```python
from build123d import *

# Parameters (mm, degrees)
SKETCH_R        = 2.8
SKETCH_R_2      = 4.3
PAD_DEPTH       = 21.5
SKETCH001_R     = 4.5
POCKET_DEPTH    = 6
SKETCH002_R     = 6.6
POCKET001_DEPTH = 9
FILLET_R        = 4


with BuildPart() as part:
    # Sketch → Pad (new body)
    with BuildSketch(Plane.XY):
        with BuildLine():
            Line((0, 0), (50, 0))
            Line((50, 0), (63.325334, 10.29541))
            ThreePointArc((63.325334, 10.29541), (67.6, 19), (63.325334, 27.70459))
            Line((50, 38), (63.325334, 27.70459))
            Line((50, 38), (0, 38))
            Line((0, 38), (-13.325334, 27.70459))
            ThreePointArc((-13.325334, 27.70459), (-17.6, 19), (-13.325334, 10.29541))
            Line((0, 0), (-13.325334, 10.29541))
        make_face()
        with Locations((5, 31)):
            Circle(SKETCH_R, mode=Mode.SUBTRACT)
        with Locations((45, 31)):
            Circle(SKETCH_R, mode=Mode.SUBTRACT)
        with Locations((45, 7)):
            Circle(SKETCH_R, mode=Mode.SUBTRACT)
        with Locations((5, 7)):
            Circle(SKETCH_R, mode=Mode.SUBTRACT)
        with Locations((-6.6, 19)):
            Circle(SKETCH_R_2, mode=Mode.SUBTRACT)
        with Locations((56.6, 19)):
            Circle(SKETCH_R_2, mode=Mode.SUBTRACT)
    extrude(amount=PAD_DEPTH)

    # Sketch001 (on Face16 of Pad) → Pocket (cut)
    with BuildSketch(Plane.XY.offset(21.5)):
        with Locations((5, 31)):
            Circle(SKETCH001_R)
        with Locations((45, 31)):
            Circle(SKETCH001_R)
        with Locations((45, 7)):
            Circle(SKETCH001_R)
        with Locations((5, 7)):
            Circle(SKETCH001_R)
    extrude(amount=-POCKET_DEPTH, mode=Mode.SUBTRACT)

    # Sketch002 (on Face4 of Pocket) → Pocket001 (cut)
    with BuildSketch(Plane(origin=(0, 0, 0), x_dir=(1, 0, 0), z_dir=(0, 0, -1))):
        with Locations((-6.6, -19)):
            Circle(SKETCH002_R)
        with Locations((56.6, -19)):
            Circle(SKETCH002_R)
    extrude(amount=-POCKET001_DEPTH, mode=Mode.SUBTRACT)

    # Fillet
    fillet_edges = [part.edges().sort_by_distance(p)[0] for p in [
        (0, 38, 10.75),
        (0, 0, 10.75),
        (50, 0, 10.75),
        (50, 38, 10.75),
    ]]
    fillet(fillet_edges, radius=FILLET_R)


solid = part.part
```
CAD build for the part. Positions are in the model's coordinates, mm. A direction names the side the tool comes from. Round coordinates to 2 decimals unless told otherwise and drop trailing zeros. Order: outer loops, then holes, each group sorted by start corner. A loop starts at its lowest first (then second) coordinate and runs counter-clockwise, first axis right, second up. Notation, with made-up numbers: (40, 55.25) - (51, 55.25) arc R23 cw to (51, 69.25) - close; hole circle Ø6 at (74, 72). An arc over 180 degrees is marked (long way). Use CSV: the item, a comma, the result in double quotes. Start each with the question number.
1) Saw through at B-B (y = 31). List the corners of the cut face in (x, z), and give its area (3 significant figures).
2) Saw through at D-D (x = 56.6). List the corners of the cut face in (y, z), and give its area (3 significant figures).
3) Saw through at A-A (z = 13.5). List the corners of the cut face in (x, y).
4) Wall check: L1, parallel to Y at x = 45, z = 7.5; L2, parallel to X at y = 19, z = 4.75; L3, parallel to X at y = 7, z = 9. Give the ranges that are in metal, low to high. Write a range as [from, to].
5) Two-plate mould, pull along Y, no slides. Class faces 4 (the cylindrical face through (4.02, 26.61, 18.54)), 5 (the flat face through (24, 19, 21.5)), 6 (the flat face through (-7.12, 5.5, 10.6)): pulls with the +Y half, pulls with the -Y half, needs draft (parallel to the pull), parting line crosses it, or undercut.
6) Pin check, flat tips, straight feed: pin 1 Ø2.5 at (x, y) = (5.5, 32.5) entering from +Z; pin 2 Ø10 at (x, z) = (-5.5, 6) entering from +Y; pin 3 Ø1 at (x, z) = (-8, 6) entering from -Y. Stop position of each tip, or through.
7) Saw through at C-C (x = 45). List the corners of the cut face in (y, z).
8) Tool access for faces 1 (the cylindrical face through (-0.503, 21.528, 4.437)), 2 (the flat face through (45, 4, 15.5)), 3 (the cylindrical face through (-2.5, 20.3, 15.2)): list every direction of +Z, -Z, +X, -X, +Y, -Y with a clear straight run to the whole face (end or side of a thin tool).
Values follow:
1,outline,"(-9.06, 0) - (2.2, 0) - (2.2, 15.5) - (0.5, 15.5) - (0.5, 21.5) - (-9.06, 21.5) - close; (7.8, 0) - (42.2, 0) - (42.2, 15.5) - (40.5, 15.5) - (40.5, 21.5) - (9.5, 21.5) - (9.5, 15.5) - (7.8, 15.5) - close; (47.8, 0) - (59.06, 0) - (59.06, 21.5) - (49.5, 21.5) - (49.5, 15.5) - (47.8, 15.5) - close"
1,area,"1,180 mm2"
2,outline,"(5.1, 0) - (12.4, 0) - (12.4, 9) - (14.7, 9) - (14.7, 21.5) - (5.1, 21.5) - close; (23.3, 9) - (25.6, 9) - (25.6, 0) - (32.9, 0) - (32.9, 21.5) - (23.3, 21.5) - close"
2,area,"371 mm2"
3,outline,"(-13.33, 10.3) - (-1.08, 0.83) arc R4 ccw to (1.37, 0) - (48.63, 0) arc R4 ccw to (51.08, 0.83) - (63.33, 10.3) arc R11 ccw to (63.33, 27.7) - (51.08, 37.17) arc R4 ccw to (48.63, 38) - (1.37, 38) arc R4 ccw to (-1.08, 37.17) - (-13.33, 27.7) arc R11 ccw to start; hole circle Ø8.6 at (-6.6, 19); hole circle Ø5.6 at (5, 7); hole circle Ø5.6 at (5, 31); hole circle Ø5.6 at (45, 7); hole circle Ø5.6 at (45, 31); hole circle Ø8.6 at (56.6, 19)"
4,L1,"y = [0, 4.2], [9.8, 28.2], [33.8, 38]"
4,L2,"x = [-17.6, -13.2], [0, 50], [63.2, 67.6]"
4,L3,"x = [-9.06, 2.2], [7.8, 42.2], [47.8, 59.06]"
5,face 4,"undercut"
5,face 5,"needs draft"
5,face 6,"pulls with the -Y half"
6,pin 1,"stops at z = 15.5"
6,pin 2,"stops at y = 37.54"
6,pin 3,"stops at y = 5.79"
7,outline,"(0, 0) - (4.2, 0) - (4.2, 15.5) - (2.5, 15.5) - (2.5, 21.5) - (0, 21.5) - close; (9.8, 0) - (28.2, 0) - (28.2, 15.5) - (26.5, 15.5) - (26.5, 21.5) - (11.5, 21.5) - (11.5, 15.5) - (9.8, 15.5) - close; (33.8, 0) - (38, 0) - (38, 21.5) - (35.5, 21.5) - (35.5, 15.5) - (33.8, 15.5) - close"
8,face 1,"-Z"
8,face 2,"+Z"
8,face 3,"+Z, -Z"
